Could you check a few things on this model? Use its own coordinates, in mm. A direction names the side the tool comes from. Give positions to 0.01 mm unless a question says otherwise; leave off trailing zeros. Order: outer loops, then holes, each group sorted by start corner. A loop starts at its lowest first (then second) coordinate and runs counter-clockwise, first axis right, second up. Notation, with made-up numbers: (68.5, -8) -> (90.5, -8) arc R14 ccw to (90.5, 19) -> close; hole circle Ø9 at (34.25, -37). An arc over 180 degrees is marked (long way). Write each question's results on one line, items separated by ' | '.
Autodesk Inventor part; units mm, degrees
ref_plane "YZ Plane" through (0, 0, 0) normal (1, 0, 0) x (0, 1, 0)
ref_plane "XZ Plane" through (0, 0, 0) normal (0, 1, 0) x (-1, 0, 0)
ref_plane "XY Plane" through (0, 0, 0) normal (0, 0, 1) x (1, 0, 0)
sketch "Sketch1" plane through (0, 0, 0) normal (0, 1, 0) x (-1, 0, 0)
  circle A0 centre (0, 0) radius 31
  circle A1 centre (0, 0) radius 33.5
  dimension "d0" = 62
  dimension "d1" = 67
extrude "Extrusion1" add sketch "Sketch1" along normal blind 23
sketch "Sketch3" plane through (0, 23, 0) normal (0, 1, 0) x (1, 0, 0)
  circle A0 centre (0, 0) radius 31
hole "Hole1" at (0, 23, 0) direction (0, -1, 0) diameter 62 end through all
sketch "Sketch4" plane through (0, 23, 0) normal (0, 1, 0) x (1, 0, 0)
  circle A0 centre (0, 0) radius 9.4443
hole "Hole2" at (0, 23, 0) direction (0, -1, 0) diameter 62 end through all
sketch "Sketch5" plane through (0, 0, 0) normal (0, -1, 0) x (1, 0, 0)
  circle A0 centre (0, 0) radius 5
  line L0 (-5, 2.5) -> (-30.9738, 2.5)
  line L1 (-5, -2.5) -> (-30.9738, -2.5)
  line L2 (-4.3301, 2.5) -> (-5, 2.5)
  line L3 (-5, -2.5) -> (-4.3301, -2.5)
  dimension "d46" = 10
extrude "Extrusion3" add sketch "Sketch5" against normal blind 23
sketch "Sketch6" plane through (0, 23, 0) normal (0, 1, 0) x (1, 0, 0)
  circle A0 centre (0, 0) radius 7.5
  dimension "d49" = 15
extrude "Extrusion4" add sketch "Sketch6" against normal blind 23
sketch "Sketch7" plane through (0, 23, 0) normal (0, 1, 0) x (1, 0, 0)
  circle A0 centre (0, 0) radius 5
  circle A1 centre (0, 0) radius 31
  circle A2 centre (0, 0) radius 7.5
  dimension "d52" = 10
extrude "Extrusion5" add sketch "Sketch7" along normal blind 11 contours A2
sketch "Sketch8" plane through (0, 0, 0) normal (0, -1, 0) x (1, 0, 0)
  circle A0 centre (0, 0) radius 7.5
  line L0 (-6.4952, 3.75) -> (-30.7723, 3.75)
  circle A1 centre (0, 0) radius 31
  line L1 (-6.4952, -3.75) -> (-30.7723, -3.75)
  line L2 (-1.9411, -7.2444) -> (-19.1077, -24.411)
  line L3 (-7.2444, -1.9411) -> (-24.411, -19.1077)
  line L4 (3.75, -6.4952) -> (3.75, -30.7723)
  line L5 (-3.75, -6.4952) -> (-3.75, -30.7723)
  line L6 (7.2444, -1.9411) -> (24.411, -19.1077)
  line L7 (1.9411, -7.2444) -> (19.1077, -24.411)
  line L8 (6.4952, 3.75) -> (30.7723, 3.75)
  line L9 (6.4952, -3.75) -> (30.7723, -3.75)
  line L10 (1.9411, 7.2444) -> (19.1077, 24.411)
  line L11 (7.2444, 1.9411) -> (24.411, 19.1077)
  line L12 (-3.75, 6.4952) -> (-3.75, 30.7723)
  line L13 (3.75, 6.4952) -> (3.75, 30.7723)
  line L14 (-7.2444, 1.9411) -> (-24.411, 19.1077)
  line L15 (-1.9411, 7.2444) -> (-19.1077, 24.411)
  point P0 (-9.0533, -3.75)
  point P1 (-3.75, -9.0533)
  point P2 (3.75, -9.0533)
  point P3 (9.0533, -3.75)
  point P4 (9.0533, 3.75)
  point P5 (3.75, 9.0533)
  point P6 (-3.75, 9.0533)
  point P7 (-9.0533, 3.75)
  dimension "d57" = 360
extrude "Extrusion6" add sketch "Sketch8" against normal blind 23 contours A0 L11 L8 A1 L9 L6 | A0 L8 L11 | L6 L9 A0 | A0 L13 L10 A1 L11 L8 | L9 L6 A1 L7 L4 A0 | A0 L10 L13 | L4 L7 A0 | A0 L15 L12 A1 L13 L10 | L7 L4 A1 L5 L2 A0 | A0 L12 L15 | L2 L5 A0 | A0 L0 L14 A1 L15 L12 | L5 L2 A1 L3 L1 A0 | A0 L14 L0 | L1 L3 A0 | A0 L3 L1 A1 L0 L14
sketch "Sketch9" plane through (0, 23, 0) normal (0, 1, 0) x (1, 0, 0)
  circle A0 centre (0, 0) radius 7.5
  circle A1 centre (0, 0) radius 7.5
  circle A2 centre (0, 0) radius 7.5
  circle A3 centre (0, 0) radius 30.9985
  point P0 (-30.7723, 3.75)
  point P1 (-30.7723, -3.75)
fillet "Fillet2" radius 2 1 edges at (-7.5, 23, 0)
properties part number "rueda de motol"
Q1. Suppose I cut it at C-C on z = 0. Please give me the cut outline in (x, y).
Here are the results:
outline: (-33.5, 0) -> (33.5, 0) -> (33.5, 23) -> (9.5, 23) arc R2 cw to (7.5, 25) -> (7.5, 34) -> (5, 34) -> (5, 23) -> (-5, 23) -> (-5, 34) -> (-7.5, 34) -> (-7.5, 25) arc R2 cw to (-9.5, 23) -> (-33.5, 23) -> close
Q2. I'm going to push flat-ended pins straight in: pin 1 Ø3 at (x, z) = (-1, -0.5) entering from +Y; pin 2 Ø12 at (y, z) = (12.5, 24.5) entering from -X; pin 3 Ø3 at (x, z) = (-6.5, -16.5) entering from -Y; pin 4 Ø17.5 at (y, z) = (7.5, -22.5) entering from +X. Where does each tip first touch, or does it pass through?
Here are the results:
pin 1: stops at y = 23 | pin 2: stops at x = -27.93 | pin 3: passes through | pin 4: stops at x = 30.55
Q3. Suppose I cut it at A-A on z = -23. Please give me the cut outline in (x, y), and give its area (3 significant figures).
Here are the results:
outline: (-24.36, 0) -> (-17.7, 0) -> (-17.7, 23) -> (-24.36, 23) -> close; (-3.75, 0) -> (3.75, 0) -> (3.75, 23) -> (-3.75, 23) -> close; (17.7, 0) -> (24.36, 0) -> (24.36, 23) -> (17.7, 23) -> close | area: 479 mm²
Q4. Suppose I cut it at D-D on x = 17. Please give me the cut outline in (y, z), and give its area (3 significant figures).
Here are the results:
outline: (0, -28.87) -> (23, -28.87) -> (23, -25.92) -> (0, -25.92) -> close; (0, -22.3) -> (23, -22.3) -> (23, -11.7) -> (0, -11.7) -> close; (0, -3.75) -> (23, -3.75) -> (23, 3.75) -> (0, 3.75) -> close; (0, 11.7) -> (23, 11.7) -> (23, 22.3) -> (0, 22.3) -> close; (0, 25.92) -> (23, 25.92) -> (23, 28.87) -> (0, 28.87) -> close | area: 796 mm²
Q5. I need wall thicknesses on line 1 along Z through (x, y) = (0, 28); line 2 along X through (y, z) = (2.5, -17); line 3 along X through (y, z) = (9, -7). Which ranges of each line are inside material? Lowest first, please.
Here are the results:
line 1: z = -7.5 to -5, 5 to 7.5 | line 2: x = -28.87 to -25.92, -22.3 to -11.7, -3.75 to 3.75, 11.7 to 22.3, 25.92 to 28.87 | line 3: x = -32.76 to -30.2, -12.3 to 12.3, 30.2 to 32.76
Q6. Suppose I cut it at B-B on x = 0. Please give me the cut outline in (y, z), and give its area (3 significant figures).
Here are the results:
outline: (0, -33.5) -> (23, -33.5) -> (23, -9.5) arc R2 cw to (25, -7.5) -> (34, -7.5) -> (34, -5) -> (23, -5) -> (23, 5) -> (34, 5) -> (34, 7.5) -> (25, 7.5) arc R2 cw to (23, 9.5) -> (23, 33.5) -> (0, 33.5) -> close | area: 1,600 mm²
Q7. Thinking about a two-plate mould opening in X: for faces 1 (the flat face through (7, 23, 8)), 2 (the cylindrical face through (-1.08, 28.42, -4.88)), 3 (the cylindrical face through (7.262, 11.339, 32.703)), which applies, +X half, -X half, draft (parallel to the pull), parting line (faces both ways), or undercut?
Here are the results:
face 1: draft | face 2: undercut | face 3: parting line
Q8. For faces 4 (the flat face through (16.625, 11.339, -11.321)), 5 (the flat face through (0, 23, 0)), which set-ups out of +Z, -Z, +X, -X, +Y, -Y let a thin tool reach every point of the face, with its end or its side?
Here are the results:
face 4: +Y, -Y | face 5: +Y
